Input: part model. Units: mm. Frame: model coordinates. A direction names the side the tool comes from. Coordinates: 2 decimals unless noted, no trailing zeros. Write each loop counter-clockwise with the first axis right and the second up, starting at its lowest first coordinate (ties: lowest second). Pieces come first, ordered by that corner, then holes. Notation, with made-up numbers: M -30.75,-33 L -12.75,-33 A10 cw -12.75,-15 Z; hole C 89.25,72 d9. An arc over 180 degrees is marked long. Answer as a JSON object with one key per item and string values. Group by question number.
from build123d import *

# Parameters (mm, degrees)
SKETCH1_W           = 679.45
SKETCH1_H           = 930.275
BOSS_EXTRUDE1_DEPTH = 30.099
SKETCH2_W           = 667.258
SKETCH2_H           = 918.083
CUT_EXTRUDE1_DEPTH  = 23.876
SKETCH3_W           = 679.45
SKETCH3_H           = 930.275
SKETCH3_W_2         = 629.666
SKETCH3_H_2         = 880.491
BOSS_EXTRUDE2_DEPTH = 0.889
SKETCH4_W           = 114.3
SKETCH4_H           = 76.2
BOSS_EXTRUDE3_DEPTH = 12.7


with BuildPart() as part:
    # Sketch1 → Boss-Extrude1 (new body)
    with BuildSketch(Plane(origin=(0, 0, 0), x_dir=(1, 0, 0), z_dir=(0, 1, 0))):
        with Locations((339.725, 465.1375)):
            Rectangle(SKETCH1_W, SKETCH1_H)
    extrude(amount=BOSS_EXTRUDE1_DEPTH)

    # Sketch2 → Cut-Extrude1 (cut)
    with BuildSketch(Plane.XZ):
        with Locations((339.725, -465.1375)):
            Rectangle(SKETCH2_W, SKETCH2_H)
    extrude(amount=-CUT_EXTRUDE1_DEPTH, mode=Mode.SUBTRACT)

    # Sketch3 → Boss-Extrude2 (add)
    with BuildSketch(Plane.XZ):
        with Locations((339.725, -465.1375)):
            Rectangle(SKETCH3_W, SKETCH3_H)
        with Locations((339.725, -465.1375)):
            Rectangle(SKETCH3_W_2, SKETCH3_H_2, mode=Mode.SUBTRACT)
    extrude(amount=-BOSS_EXTRUDE2_DEPTH)

    # Sketch4 → Boss-Extrude3 (add)
    with BuildSketch(Plane.XZ.offset(-23.876)):
        with Locations((339.725, -828.675)):
            Rectangle(SKETCH4_W, SKETCH4_H)
    extrude(amount=BOSS_EXTRUDE3_DEPTH)


solid = part.part
Q1. Section D-D, the plane x = 568. Return the cut outline in (y, z) (3 decimals).
Q2. Pin query (flat end, axial travel): pin 1 Ø1.5 at (x, z) = (528.5, -259) entering from -Y. Return the tip coordinate at first contact, or that it passes through.
Q3. Draft query along Z for faces 3 (the flat face through (335, 15, -930.275)), 4 (the flat face through (339, 11.176, -828)), 5 (the flat face through (335, 30.099, -472)). Return one class per face: released by +Z, released by -Z, zero draft, split by the parting line, or undercut.
Q4. Section C-C, the plane z = -498. Return the cut outline in (x, y), and give its area (3 significant figures).
Q5. Section A-A, the plane y = 19. Return the cut outline in (x, z) (3 decimals), and give its area (3 significant figures).
Q6. Section B-B, the plane x = 380. Return the cut outline in (y, z) (3 decimals), and give its area (3 significant figures).
Q7. Line query: line 1 (Z direction, x = 220.5, y = 10.5) (3 decimals); line 2 (X direction, y = 1.5, z = -413); line 3 (Y direction, x = 587.5, z = -338). Output: solid intervals per line, ascending. Write a range as from..to.
Q8. Access query for faces 1 (the flat face through (335, 15, 0)), 2 (the flat face through (673.354, 12, -472)). Directions: +Z, -Z, +X, -X, +Y, -Y. A direction counts if a zero-diameter tool reaches every point of the face in a straight line with its end or side. Return the directions, or none.
Filled in:
{
 "1": {"outline": "M 0,-930.275 L 30.099,-930.275 L 30.099,0 L 0,0 L 0,-24.892 L 0.889,-24.892 L 0.889,-6.096 L 23.876,-6.096 L 23.876,-924.179 L 0.889,-924.179 L 0.889,-905.383 L 0,-905.383 Z"},
 "2": {"pin 1": "y = 23.88"},
 "3": {"face 3": "released by -Z", "face 4": "undercut", "face 5": "zero draft"},
 "4": {"outline": "M 0,0 L 24.89,0 L 24.89,0.89 L 6.1,0.89 L 6.1,23.88 L 673.35,23.88 L 673.35,0.89 L 654.56,0.89 L 654.56,0 L 679.45,0 L 679.45,30.1 L 0,30.1 Z", "area": "4,550 mm^2"},
 "5": {"outline": "M 0,-930.275 L 679.45,-930.275 L 679.45,0 L 0,0 Z; M 282.575,-866.775 L 396.875,-866.775 L 396.875,-790.575 L 282.575,-790.575 Z; hole M 6.096,-924.179 L 673.354,-924.179 L 673.354,-6.096 L 6.096,-6.096 Z", "area": "28,200 mm^2"},
 "6": {"outline": "M 0,-930.275 L 30.099,-930.275 L 30.099,0 L 0,0 L 0,-24.892 L 0.889,-24.892 L 0.889,-6.096 L 23.876,-6.096 L 23.876,-790.575 L 11.176,-790.575 L 11.176,-866.775 L 23.876,-866.775 L 23.876,-924.179 L 0.889,-924.179 L 0.889,-905.383 L 0,-905.383 Z", "area": "7,080 mm^2"},
 "7": {"line 1": "-930.275..-924.179, -6.096..0", "line 2": "0..6.1, 673.35..679.45", "line 3": "23.88..30.1"},
 "8": {"face 1": "+Z, +X, -X, +Y, -Y", "face 2": "none"}
}
